from build123d import *

# Parameters (mm, degrees)
SKETCH1_W               = 38
SKETCH1_H               = 21
SKETCH1_R               = 1.4
BOSS_EXTRUDE1_DEPTH     = 2
CUT_EXTRUDE1_DEPTH      = 104.179455
CUT_EXTRUDE1_DEPTH_BACK = 104.179455
SKETCH3_R               = 11.1
CUT_EXTRUDE2_DEPTH      = 104.179455
CUT_EXTRUDE2_DEPTH_BACK = 104.179455
SKETCH4_R               = 2.5
BOSS_EXTRUDE2_START     = -12.28
BOSS_EXTRUDE2_OUTLINE_R = 1.4
BOSS_EXTRUDE2_DEPTH     = 10.28
CUT_EXTRUDE3_START      = -10.28
SKETCH6_W               = 42
SKETCH6_H               = 42
SKETCH6_R               = 1.4
CUT_EXTRUDE3_DEPTH      = 10.28
CUT_EXTRUDE4_DEPTH      = 110.866639
CUT_EXTRUDE4_DEPTH_BACK = 110.866639
SKETCH7_W               = 17
SKETCH7_H               = 10.28
FILLET1_R               = 1


# Read off the part's stored shape, not the designer's step: Boss-Extrude2
with BuildPart() as part:
    # Sketch1 → Boss-Extrude1 (new body)
    # profile 1 of 4: a face of its own
    with BuildSketch(Plane(origin=(0, 0, 0), x_dir=(1, 0, 0), z_dir=(0, 1, 0))):
        with Locations((40, 10.5)):
            Rectangle(SKETCH1_W, SKETCH1_H)
    # profile 2 of 4: a face of its own
    with BuildSketch(Plane(origin=(0, 0, 0), x_dir=(1, 0, 0), z_dir=(0, 1, 0))):
        Polygon((21, -21), (21, 0), (21, 21), (-21, 21), (-21, -21), align=None)
        with Locations(Location((-15.5, -15.5, 0), (0, 0, 270))):
            Circle(SKETCH1_R, mode=Mode.SUBTRACT)
        with Locations(Location((15.5, -15.5, 0), (0, 0, 270))):
            Circle(SKETCH1_R, mode=Mode.SUBTRACT)
        with Locations(Location((-15.5, 15.5, 0), (0, 0, 270))):
            Circle(SKETCH1_R, mode=Mode.SUBTRACT)
        with Locations(Location((15.5, 15.5, 0), (0, 0, 270))):
            Circle(SKETCH1_R, mode=Mode.SUBTRACT)
    # profile 3 of 4: a face of its own
    with BuildSketch(Plane(origin=(0, 0, 0), x_dir=(1, 0, 0), z_dir=(0, 1, 0))):
        with Locations((40, -10.5)):
            Rectangle(SKETCH1_W, SKETCH1_H)
    # profile 4 of 4: a face of its own
    with BuildSketch(Plane(origin=(0, 0, 0), x_dir=(1, 0, 0), z_dir=(0, 1, 0))):
        Polygon((59, 21), (59, 0), (59, -21), (101, -21), (101, 21), align=None)
        with Locations(Location((64.5, -15.5, 0), (0, 0, 270))):
            Circle(SKETCH1_R, mode=Mode.SUBTRACT)
        with Locations(Location((95.5, -15.5, 0), (0, 0, 270))):
            Circle(SKETCH1_R, mode=Mode.SUBTRACT)
        with Locations(Location((64.5, 15.5, 0), (0, 0, 270))):
            Circle(SKETCH1_R, mode=Mode.SUBTRACT)
        with Locations(Location((95.5, 15.5, 0), (0, 0, 270))):
            Circle(SKETCH1_R, mode=Mode.SUBTRACT)
    extrude(amount=BOSS_EXTRUDE1_DEPTH)

    # Sketch3 → Cut-Extrude1 (cut, two sides: drawn at the far end of the back side and taken through both)
    with BuildSketch(Plane(origin=(0, 2, 0), x_dir=(1, 0, 0), z_dir=(0, 1, 0)).offset(-CUT_EXTRUDE1_DEPTH_BACK)):
        with Locations(Location((80, 0, 0), (0, 0, 270))):
            Circle(SKETCH3_R)
        with Locations(Location((0, 0, 0), (0, 0, 270))):
            Circle(SKETCH3_R)
    extrude(amount=CUT_EXTRUDE1_DEPTH + CUT_EXTRUDE1_DEPTH_BACK, mode=Mode.SUBTRACT)

    # Sketch4 → Cut-Extrude2 (cut, two sides: drawn at the far end of the back side and taken through both)
    with BuildSketch(Plane(origin=(0, 2, 0), x_dir=(1, 0, 0), z_dir=(0, 1, 0)).offset(-CUT_EXTRUDE2_DEPTH_BACK)):
        with Locations(Location((40, 0, 0), (0, 0, 270))):
            Circle(SKETCH4_R)
    extrude(amount=CUT_EXTRUDE2_DEPTH + CUT_EXTRUDE2_DEPTH_BACK, mode=Mode.SUBTRACT)


with BuildPart() as boss_extrude2_tool:
    # Boss-Extrude2 outline → Boss-Extrude2 (new body)
    with BuildSketch(Plane(origin=(0, 2, 0), x_dir=(1, 0, 0), z_dir=(0, 1, 0)).offset(BOSS_EXTRUDE2_START)):
        with BuildLine():
            Line((-21, -21), (40, -21))
            Line((40, -21), (40, -2.5))
            ThreePointArc((40, -2.5), (37.5, 0), (40, 2.5))
            Line((40, 2.5), (40, 21))
            Line((40, 21), (-21, 21))
            Line((-21, 21), (-21, -21))
        make_face()
        with Locations((-15.5, -15.5)):
            Circle(BOSS_EXTRUDE2_OUTLINE_R, mode=Mode.SUBTRACT)
        with Locations((15.5, -15.5)):
            Circle(BOSS_EXTRUDE2_OUTLINE_R, mode=Mode.SUBTRACT)
        with BuildLine():
            add(Edge.make_bspline(
                [(0, -11.1), (-0.726845, -11.100027), (-2.180374, -10.961006), (-4.27463, -10.319187), (-6.209027, -9.292142), (-7.898295, -7.897803), (-9.292338, -6.208724), (-10.319432, -4.274073), (-10.960977, -2.180089), (-11.169529, 0.000347), (-10.960906, 2.180445), (-10.319167, 4.274715), (-9.292137, 6.209025), (-7.897804, 7.898295), (-6.208724, 9.292338), (-4.274073, 10.319432), (-2.180089, 10.960977), (0.000347, 11.169529), (2.180445, 10.960906), (4.274715, 10.319167), (6.209025, 9.292137), (7.898295, 7.897804), (9.292338, 6.208724), (10.319432, 4.274073), (10.960977, 2.180089), (11.169529, -0.000347), (10.960906, -2.180445), (10.319167, -4.274715), (9.292137, -6.209025), (7.897805, -7.898297), (6.208722, -9.292332), (4.274158, -10.319412), (2.180159, -10.960877), (0.726667, -11.099973), (0, -11.1)],
                knots=[0, 0, 0, 0, 0.031254, 0.0625, 0.093758, 0.125, 0.156258, 0.1875, 0.218758, 0.25, 0.281258, 0.3125, 0.343758, 0.375, 0.406258, 0.4375, 0.468758, 0.5, 0.531258, 0.5625, 0.593758, 0.625, 0.656258, 0.6875, 0.718758, 0.75, 0.781258, 0.8125, 0.843758, 0.875, 0.906258, 0.9375, 0.968754, 1, 1, 1, 1], degree=3))
        make_face(mode=Mode.SUBTRACT)
        with Locations((-15.5, 15.5)):
            Circle(BOSS_EXTRUDE2_OUTLINE_R, mode=Mode.SUBTRACT)
        with Locations((15.5, 15.5)):
            Circle(BOSS_EXTRUDE2_OUTLINE_R, mode=Mode.SUBTRACT)
    extrude(amount=BOSS_EXTRUDE2_DEPTH)


with BuildPart() as part_1:
    add(part.part)


with BuildPart() as part_2:
    # Boss-Extrude2: joined with boss_extrude2_tool
    add(part_1.part.fuse(boss_extrude2_tool.part, tol=0.00001))

    # Sketch6 → Cut-Extrude3 (cut)
    with BuildSketch(Plane(origin=(0, 2, 0), x_dir=(1, 0, 0), z_dir=(0, 1, 0)).offset(CUT_EXTRUDE3_START)):
        Rectangle(SKETCH6_W, SKETCH6_H)
        with Locations(Location((15.5, 15.5, 0), (0, 0, 270))):
            Circle(SKETCH6_R, mode=Mode.SUBTRACT)
        with Locations(Location((-15.5, 15.5, 0), (0, 0, 270))):
            Circle(SKETCH6_R, mode=Mode.SUBTRACT)
        with Locations(Location((-15.5, -15.5, 0), (0, 0, 270))):
            Circle(SKETCH6_R, mode=Mode.SUBTRACT)
        with Locations(Location((15.5, -15.5, 0), (0, 0, 270))):
            Circle(SKETCH6_R, mode=Mode.SUBTRACT)
    extrude(amount=CUT_EXTRUDE3_DEPTH, mode=Mode.SUBTRACT)

    # Sketch7 → Cut-Extrude4 (cut, two sides: drawn at the far end of the back side and taken through both)
    with BuildSketch(Plane.XY.offset(21).offset(-CUT_EXTRUDE4_DEPTH_BACK)):
        with Locations((31.5, -5.14)):
            Rectangle(SKETCH7_W, SKETCH7_H)
    extrude(amount=CUT_EXTRUDE4_DEPTH + CUT_EXTRUDE4_DEPTH_BACK, mode=Mode.SUBTRACT)

    # Fillet1
    fillet1_edges = [part_2.edges().sort_by_distance(p)[0] for p in [
        (21, -8.28, 0),
        (21, 2, 0),
        (23, 0, 0),
    ]]
    fillet(fillet1_edges, radius=FILLET1_R)


solid = part_2.part
Design review of the part built by this model. Coordinates are the model's own, in mm. A direction names the side the tool comes from. Round coordinates to 2 decimals unless told otherwise and drop trailing zeros. Write each loop counter-clockwise with the first axis right and the second up, starting at its lowest first coordinate (ties: lowest second). Pieces come first, ordered by that corner, then holes. Notation, with made-up numbers: M 14,36.5 L 56,36.5 A21 cw 56,69.5 Z; hole C -6.5,1.25 d11. An arc over 180 degrees is marked long. One line per item, written item: value. Start each with the question number.
1. Take a section at C-C on z = -18. State the section outline as (x, y) points.
2. Take a section at D-D on x = 95.5. State the section outline as (y, z) points, then the cut area to 3 significant figures.
3. For faces 4 (the face through (62, 0, 0)), 5 (the face through (-10, -8.28, -10)), 6 (the face through (-21, -9, 0)), list the 3-axis set-ups (+Z, -Z, +X, -X, +Y, -Y) from which the entire face can be reached by the end or side of a thin tool; tool diameter is ignored.
4. To check wall thickness, follow probe 1 along Z at (x, y) = (95.5, 1.25); probe 2 along X at (y, z) = (1.2, 15.5); probe 3 along X at (y, z) = (0.6, 0). State the ranges of each line that lie inside material, in increasing order. Write a range as from..to.
5. Draft analysis for pull direction Z (two halves, no side actions). For faces 1 (the face through (69.164, 0.986, -2.406)), 2 (the face through (21, -3, 0)), 3 (the face through (35.2, 0.4, 21)), state which applies: pulls with the +Z half, pulls with the -Z half, needs draft (parallel to the pull), parting line crosses it, or undercut.
6. Take a section at A-A on x = 40. State the section outline as (y, z) points.
7. Take a section at B-B on z = 15.5. State the section outline as (x, y) points, then the cut area to 3 significant figures.
8. Clearance check with flat-ended pins moving along their axes: P1, Ø3, axis at x = 95.5, z = -15.5, coming from the -Y side; P2, Ø4, axis at y = -2, z = 2.5, coming from the -X side; P3, Ø1, axis at y = -4, z = 2.5, coming from the +X side. State where each tip first meets the part, or that it passes through.
Computed:
1. outline: M -21,-10.28 L 23,-10.28 L 23,-1 A1 cw 24,0 L 101,0 L 101,2 L 22,2 A1 ccw 21,1 L 21,-7.28 A1 cw 20,-8.28 L -21,-8.28 Z
2. outline: M 0,-21 L 2,-21 L 2,-16.9 L 0,-16.9 Z; M 0,-14.1 L 2,-14.1 L 2,14.1 L 0,14.1 Z; M 0,16.9 L 2,16.9 L 2,21 L 0,21 Z
2. area: 72.8 mm²
3. face 4: +Z, -Z, +X, -Y
3. face 5: +Z, -Z, -X, +Y
3. face 6: +Z, -Z, -X, +Y, -Y
4. probe 1: z = -21..-16.9, -14.1..14.1, 16.9..21
4. probe 2: x = 21.02..63.1, 65.9..94.1, 96.9..101
4. probe 3: x = 21..37.5, 42.5..68.9, 91.1..101
5. face 1: undercut
5. face 2: needs draft
5. face 3: pulls with the +Z half
6. outline: M 0,-21 L 2,-21 L 2,-2.5 L 0,-2.5 Z; M 0,2.5 L 2,2.5 L 2,21 L 0,21 Z
7. outline: M -21,-10.28 L -16.9,-10.28 L -16.9,-8.28 L -21,-8.28 Z; M -14.1,-10.28 L 14.1,-10.28 L 14.1,-8.28 L -14.1,-8.28 Z; M 16.9,-10.28 L 23,-10.28 L 23,-1 A1 cw 24,0 L 63.1,0 L 63.1,2 L 22,2 A1 ccw 21,1 L 21,-7.28 A1 cw 20,-8.28 L 16.9,-8.28 Z; M 65.9,0 L 94.1,0 L 94.1,2 L 65.9,2 Z; M 96.9,0 L 101,0 L 101,2 L 96.9,2 Z
7. area: 242 mm²
8. P1: stops at y = 0
8. P2: stops at x = 21
8. P3: stops at x = 23
